Could you check a few things on this drawing? It's one solid part, dimensions in mm from its lowest x, y, z. Give positions to 0.01 mm unless a question says otherwise; leave off trailing zeros. Order: outer loops, then holes, each group sorted by start corner. A loop starts at its lowest first (then second) coordinate and runs counter-clockwise, first axis right, second up. Notation, with made-up numbers: (55.5, 65) -> (109.5, 65) arc R9 ccw to (109.5, 71) -> close; hole circle Ø9 at (33, 38.25). An arc over 180 degrees is marked (long way). Write each question's results on one line, items separated by ' | '.
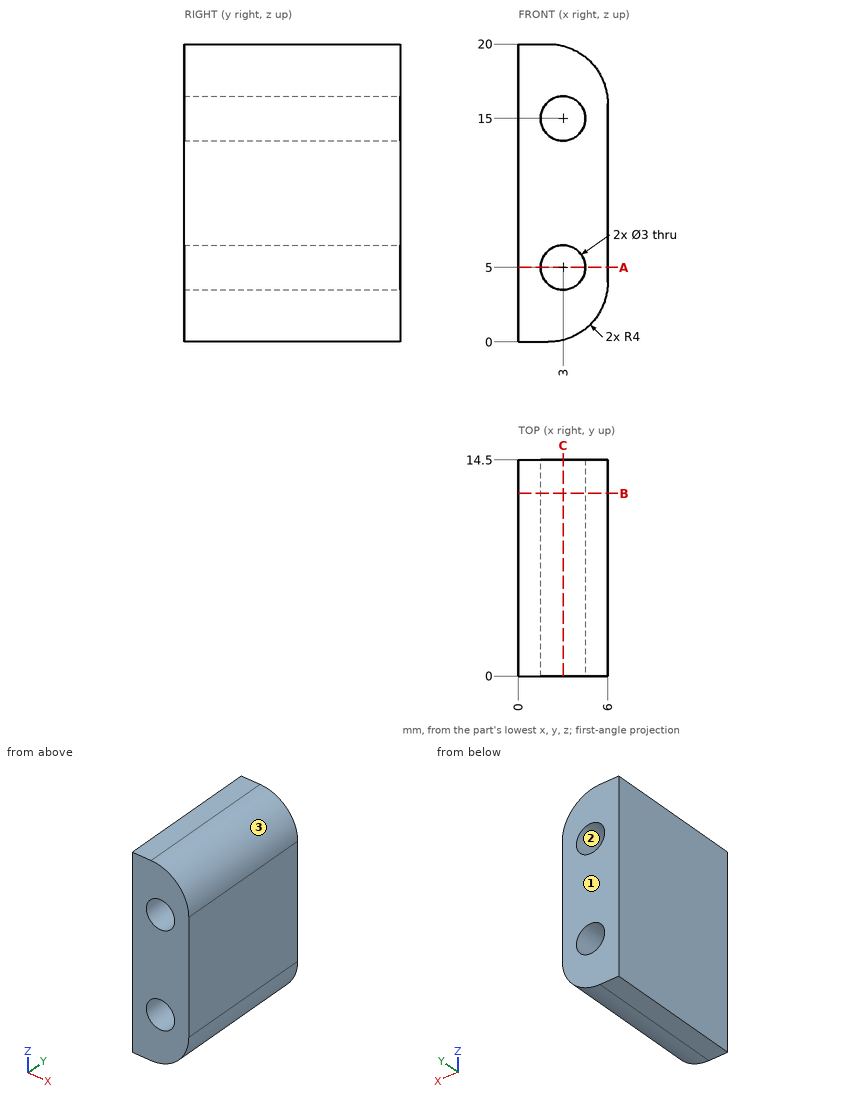
Q1. I need wall thicknesses on line 1 along Z through (x, y) = (3, 10.25); line 2 along X through (y, z) = (8.75, 15); line 3 along Z through (x, y) = (2.25, 2). Which ranges of each line are inside material? Lowest first, please.
Here are the results:
line 1: z = 0.13 to 3.5, 6.5 to 13.5, 16.5 to 19.87 | line 2: x = 0 to 1.5, 4.5 to 6 | line 3: z = 0.01 to 3.7, 6.3 to 13.7, 16.3 to 19.99
Q2. Suppose I cut it at C-C on x = 3. Please give me the cut outline in (y, z).
Here are the results:
outline: (0, 0.13) -> (14.5, 0.13) -> (14.5, 3.5) -> (0, 3.5) -> close; (0, 6.5) -> (14.5, 6.5) -> (14.5, 13.5) -> (0, 13.5) -> close; (0, 16.5) -> (14.5, 16.5) -> (14.5, 19.87) -> (0, 19.87) -> close
Q3. Thinking about a two-plate mould opening in Z: for the marked faces 1, 2 and 3, which applies, +Z half, -Z half, draft (parallel to the pull), parting line (faces both ways), or undercut?
Here are the results:
face 1: draft | face 2: undercut | face 3: +Z half
Q4. I'm going to push flat-ended pins straight in: pin 1 Ø1.5 at (x, y) = (4.5, 13) entering from -Z; pin 2 Ø3 at (x, z) = (2, 6) entering from -Y. Where does each tip first touch, or does it pass through?
Here are the results:
pin 1: stops at z = 0.4 | pin 2: stops at y = 0
Q5. Suppose I cut it at B-B on y = 12.25. Please give me the cut outline in (x, z).
Here are the results:
outline: (0, 0) -> (2, 0) arc R4 ccw to (6, 4) -> (6, 16) arc R4 ccw to (2, 20) -> (0, 20) -> close; hole circle Ø3 at (3, 5); hole circle Ø3 at (3, 15)
Q6. Suppose I cut it at A-A on z = 5. Please give me the cut outline in (x, y).
Here are the results:
outline: (0, 0) -> (1.5, 0) -> (1.5, 14.5) -> (0, 14.5) -> close; (4.5, 0) -> (6, 0) -> (6, 14.5) -> (4.5, 14.5) -> close
